Work out the finished part from the listing and answer in its coordinate system (mm). Face numbers are marked on the shaded views. A direction names the side the tool comes from. Give positions to 0.01 mm unless a question says otherwise; leave off trailing zeros. Loops run counter-clockwise (first coordinate to the right, second up) from the corner with the lowest first, then second, coordinate; pieces in that order, holes last. Notation, with made-up numbers: M 15.25,-19.5 L 20.25,-19.5 A12 ccw 20.25,-8.5 Z; hole C -5.75,72.5 d10. An arc over 180 degrees is marked long. Answer in a Markdown table with one row per item. Add a question column.
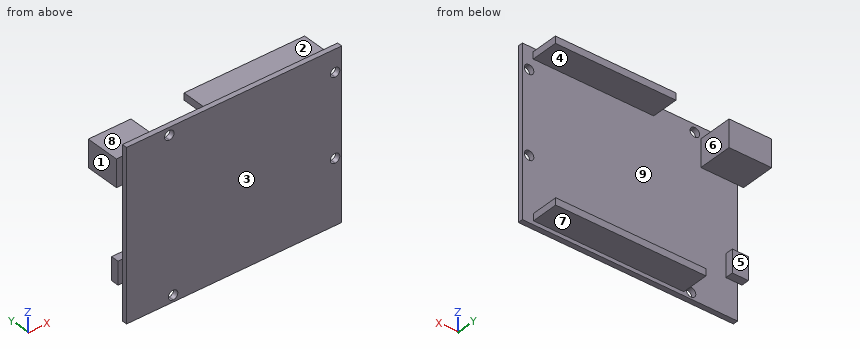
from build123d import *

# Parameters (mm, degrees)
SKETCH1_W                  = 68
SKETCH1_H                  = 53
BOSS_EXTRUDE1_DEPTH        = 1.6
M2_5_CLEARANCE_SLOT1_DEPTH = 1.6
SKETCH4_W                  = 47.5
SKETCH4_H                  = 2.2
SKETCH4_W_2                = 38.1
BOSS_EXTRUDE2_DEPTH        = 8.6
SKETCH5_W                  = 13.5
SKETCH5_H                  = 8.6
BOSS_EXTRUDE3_DEPTH        = 10.9
SKETCH6_W                  = 5.1
SKETCH6_H                  = 7.2
BOSS_EXTRUDE4_DEPTH        = 2.5


# Read off the part's stored shape, not the designer's step: M2.5 Clearance Slot1
with BuildPart() as part:
    # Sketch1 → Boss-Extrude1 (new body)
    with BuildSketch(Plane(origin=(0, 0, 0), x_dir=(1, 0, 0), z_dir=(0, 1, 0))):
        with Locations((34, 26.5)):
            Rectangle(SKETCH1_W, SKETCH1_H)
    extrude(amount=BOSS_EXTRUDE1_DEPTH)

    # M2.5 Clearance Slot1 outline → M2.5 Clearance Slot1 (cut)
    with BuildSketch(Plane(origin=(0, 0, 0), x_dir=(1, 0, 0), z_dir=(0, 1, 0))):
        with BuildLine():
            Line((14.65, 49.45), (14.75, 49.45))
            ThreePointArc((14.75, 49.45), (16.2, 50.9), (14.75, 52.35))
            Line((14.75, 52.35), (14.65, 52.35))
            ThreePointArc((14.65, 52.35), (13.2, 50.9), (14.65, 49.45))
        make_face()
        with BuildLine():
            Line((65.85, 31.35), (65.95, 31.35))
            ThreePointArc((65.95, 31.35), (67.4, 32.8), (65.95, 34.25))
            Line((65.95, 34.25), (65.85, 34.25))
            ThreePointArc((65.85, 34.25), (64.4, 32.8), (65.85, 31.35))
        make_face()
        with BuildLine():
            Line((65.85, 5.55), (65.95, 5.55))
            ThreePointArc((65.95, 5.55), (67.4, 7), (65.95, 8.45))
            Line((65.95, 8.45), (65.85, 8.45))
            ThreePointArc((65.85, 8.45), (64.4, 7), (65.85, 5.55))
        make_face()
        with BuildLine():
            Line((13.45, 0.95), (13.55, 0.95))
            ThreePointArc((13.55, 0.95), (15, 2.4), (13.55, 3.85))
            Line((13.55, 3.85), (13.45, 3.85))
            ThreePointArc((13.45, 3.85), (12, 2.4), (13.45, 0.95))
        make_face()
    extrude(amount=M2_5_CLEARANCE_SLOT1_DEPTH, mode=Mode.SUBTRACT)

    # Sketch4 → Boss-Extrude2 (add)
    with BuildSketch(Plane(origin=(0, 1.6, 0), x_dir=(1, 0, 0), z_dir=(0, 1, 0))):
        with Locations((40.75, 50.7)):
            Rectangle(SKETCH4_W, SKETCH4_H)
        with Locations((45.55, 2.2)):
            Rectangle(SKETCH4_W_2, SKETCH4_H)
    extrude(amount=BOSS_EXTRUDE2_DEPTH)

    # Sketch5 → Boss-Extrude3 (add)
    with BuildSketch(Plane(origin=(0, 1.6, 0), x_dir=(1, 0, 0), z_dir=(0, 1, 0))):
        with Locations((4.85, 7.8)):
            Rectangle(SKETCH5_W, SKETCH5_H)
    extrude(amount=BOSS_EXTRUDE3_DEPTH)

    # Sketch6 → Boss-Extrude4 (add)
    with BuildSketch(Plane(origin=(0, 1.6, 0), x_dir=(1, 0, 0), z_dir=(0, 1, 0))):
        with Locations((1.15, 38)):
            Rectangle(SKETCH6_W, SKETCH6_H)
    extrude(amount=BOSS_EXTRUDE4_DEPTH)


solid = part.part
(1) Section C-C, the plane x = 24 is taken. Determine the outline of the cut face in (y, z), and give its area (3 significant figures).
(2) Section D-D, the plane z = -2.4 is taken. Determine the outline of the cut face in (x, y).
(3) The mould has two halves that part along Z. Classify the marked faces 6, 7, 8 and 9: pulls with the +Z half, pulls with the -Z half, needs draft (parallel to the pull), parting line crosses it, or undercut.
(4) Consider line 1 along Z through (x, y) = (52, 5.25); line 2 along X through (y, z) = (0.75, -5); line 3 along Y through (x, z) = (26.5, -33.5). Determine where each line is inside the solid, lowest interval first. Write a range as from..to.
(5) Section B-B, the plane y = 6.25 is taken. Determine the outline of the cut face in (x, z), and give its area (3 significant figures).
(6) Which of the six approach directions +Z, -Z, +X, -X, +Y, -Y give full straight-line access (tool end or side, diameter ignored) to the marked faces 1, 2, 3, 4 and 5?
(7) Section A-A, the plane z = -32.8 is taken. Determine the outline of the cut face in (x, y).
(8) Each of these flat-tipped pins is pushed along its axis until it touches: P1, Ø12, axis at x = 36.5, z = -13, coming from the +Y side; P2, Ø1.1, axis at y = 6, z = -50.5, coming from the +X side; P3, Ø7, axis at x = 32, y = 7.5, coming from the -Z side. Where does it stop, or does it pass through?
Numbers:
| question | item | result |
|---|---|---|
| 1 | outline | M 0,-53 L 1.6,-53 L 1.6,-51.8 L 10.2,-51.8 L 10.2,-49.6 L 1.6,-49.6 L 1.6,0 L 0,0 Z |
| 1 | area | 104 mm² |
| 2 | outline | M 0,0 L 12,0 L 12,1.6 L 0,1.6 Z; M 15,0 L 68,0 L 68,1.6 L 64.6,1.6 L 64.6,10.2 L 26.5,10.2 L 26.5,1.6 L 15,1.6 Z |
| 3 | face 6 | needs draft |
| 3 | face 7 | pulls with the -Z half |
| 3 | face 8 | pulls with the +Z half |
| 3 | face 9 | undercut |
| 4 | line 1 | z = -51.8..-49.6, -3.3..-1.1 |
| 4 | line 2 | x = 0..68 |
| 4 | line 3 | y = 0..1.6 |
| 5 | outline | M -1.9,-12.1 L 11.6,-12.1 L 11.6,-3.5 L -1.9,-3.5 Z; M 17,-51.8 L 64.5,-51.8 L 64.5,-49.6 L 17,-49.6 Z; M 26.5,-3.3 L 64.6,-3.3 L 64.6,-1.1 L 26.5,-1.1 Z |
| 5 | area | 304 mm² |
| 6 | face 1 | +Z, -Z, -X, +Y, -Y |
| 6 | face 2 | +Z, +X, -X, +Y |
| 6 | face 3 | +Z, -Z, +X, -X, -Y |
| 6 | face 4 | +X, -X, +Y |
| 6 | face 5 | -Z, +X, -X, +Y |
| 7 | outline | M 0,0 L 64.4,0 L 64.4,1.6 L 0,1.6 Z; M 67.4,0 L 68,0 L 68,1.6 L 67.4,1.6 Z |
| 8 | P1 | stops at y = 1.6 |
| 8 | P2 | stops at x = 64.5 |
| 8 | P3 | stops at z = -51.8 |
